Verification items for the finished model (mm, model axes). A direction names the side the tool comes from. Coordinates: 2 decimals unless noted, no trailing zeros. Order: outer loops, then holes, each group sorted by start corner. A loop starts at its lowest first (then second) coordinate and runs counter-clockwise, first axis right, second up. Notation, with made-up numbers: (-14.5, 21) - (36.5, 21) arc R12 cw to (36.5, 27) - close; hole circle Ø5 at (-1.5, 42). An arc over 180 degrees is marked (long way). One line per question, with ' | ' between items. Start each with the question number.
from build123d import *

# Parameters (mm, degrees)
SKETCH1_W               = 22.65
SKETCH1_H               = 31.12
PCB_DEPTH               = 1.3
SKETCH2_W               = 9.55
SKETCH2_H               = 7.3
IO_CONNECTOR_DEPTH      = 4.2
SKETCH3_W               = 3
SKETCH3_H               = 3.5
ANTENNA_CONNECTOR_DEPTH = 2
SKETCH15_W              = 3
SKETCH15_H              = 3.9
BUTTON_BASE_DEPTH       = 1.3
SKETCH16_R              = 0.9
BUTTON_TIP_DEPTH        = 0.8
SKETCH17_W              = 6.157933233
SKETCH17_H              = 6.029642957
SKETCH17_W_2            = 3.353874351
SKETCH17_H_2            = 3.005657888
SKETCH17_W_3            = 3.060639434
SKETCH17_H_3            = 1.576137673
SKETCH17_H_4            = 1.612792038
SKETCH17_W_4            = 3.201337113
SKETCH17_H_5            = 3.020980094
LOW_CHIPS_DEPTH         = 1
SKETCH18_W              = 6.492852738
SKETCH18_H              = 7.038252368
HIGH_CHIPS_DEPTH        = 2.7
SKETCH23_W              = 2
SKETCH23_H              = 0.8
LEDS_DEPTH              = 0.5
CORNERS_R               = 1
CUT_EXTRUDE1_REACH      = 24.031
SKETCH24_W              = 1.1
SKETCH24_H              = 2.5


with BuildPart() as part:
    # Sketch1 → PCB (new body)
    with BuildSketch(Plane(origin=(0, 0, 0), x_dir=(1, 0, 0), z_dir=(0, 1, 0))):
        Rectangle(SKETCH1_W, SKETCH1_H)
    extrude(amount=PCB_DEPTH)

    # Sketch2 → IO connector (add)
    with BuildSketch(Plane(origin=(0, 1.3, 0), x_dir=(1, 0, 0), z_dir=(0, 1, 0))):
        with Locations((6.55, -14.41)):
            Rectangle(SKETCH2_W, SKETCH2_H)
    extrude(amount=IO_CONNECTOR_DEPTH)

    # Sketch3 → Antenna connector (add)
    with BuildSketch(Plane(origin=(0, 1.3, 0), x_dir=(1, 0, 0), z_dir=(0, 1, 0))):
        with Locations((-8.025, 13.81)):
            Rectangle(SKETCH3_W, SKETCH3_H)
    extrude(amount=ANTENNA_CONNECTOR_DEPTH)

    # Sketch15 → Button base (add)
    with BuildSketch(Plane(origin=(0, 1.3, 0), x_dir=(1, 0, 0), z_dir=(0, 1, 0))):
        with Locations((-9.325, -12.41)):
            Rectangle(SKETCH15_W, SKETCH15_H)
    extrude(amount=BUTTON_BASE_DEPTH)

    # Sketch16 → Button tip (add)
    with BuildSketch(Plane(origin=(0, 2.6, 0), x_dir=(1, 0, 0), z_dir=(0, 1, 0))):
        with Locations(Location((-9.325, -12.41, 0), (0, 0, 90))):
            Circle(SKETCH16_R)
    extrude(amount=BUTTON_TIP_DEPTH)

    # Sketch17 → Low chips (add)
    with BuildSketch(Plane(origin=(0, 1.3, 0), x_dir=(1, 0, 0), z_dir=(0, 1, 0))):
        with Locations((-2.078363242, 3.759055692)):
            Rectangle(SKETCH17_W, SKETCH17_H)
        with Locations((-7.585681506, 8.185070203)):
            Rectangle(SKETCH17_W_2, SKETCH17_H_2)
        with Locations((9.825141625, 11.942142563)):
            Rectangle(SKETCH17_W_3, SKETCH17_H_3)
        with Locations((5.829815896, 11.044110633)):
            Rectangle(SKETCH17_W_3, SKETCH17_H_4)
        with Locations((-4.917111521, -2.959047528)):
            Rectangle(SKETCH17_W_4, SKETCH17_H_5)
    extrude(amount=LOW_CHIPS_DEPTH)

    # Sketch18 → High chips (add)
    with BuildSketch(Plane(origin=(0, 1.3, 0), x_dir=(1, 0, 0), z_dir=(0, 1, 0))):
        with Locations((8.086930252, -1.973636887)):
            Rectangle(SKETCH18_W, SKETCH18_H)
    extrude(amount=HIGH_CHIPS_DEPTH)

    # Sketch23 → LEDs (add)
    with BuildSketch(Plane(origin=(0, 1.3, 0), x_dir=(1, 0, 0), z_dir=(0, 1, 0))):
        with Locations((-9.725, -8.36)):
            Rectangle(SKETCH23_W, SKETCH23_H)
        with Locations((-9.725, -6.91)):
            Rectangle(SKETCH23_W, SKETCH23_H)
    extrude(amount=LEDS_DEPTH)

    # Corners
    corners_edges = [part.edges().sort_by_distance(p)[0] for p in [
        (11.325, 0.65, 15.56),
        (-11.325, 0.65, 15.56),
        (-11.325, 0.65, -15.56),
        (11.325, 0.65, -15.56),
    ]]
    fillet(corners_edges, radius=CORNERS_R)

    # Sketch24 → Cut-Extrude1 (cut, up to next)
    with BuildSketch(Plane(origin=(0, 5.5, 0), x_dir=(1, 0, 0), z_dir=(0, 1, 0)), mode=Mode.PRIVATE) as cut_extrude1_sk1:
        with Locations((10.775, -16.81)):
            Rectangle(SKETCH24_W, SKETCH24_H)
    cut_extrude1_tool1 = extrude(cut_extrude1_sk1.sketch, amount=-CUT_EXTRUDE1_REACH, mode=Mode.PRIVATE) & part.part
    # Sketch24 → Cut-Extrude1 (cut, up to next)
    with BuildSketch(Plane(origin=(0, 5.5, 0), x_dir=(1, 0, 0), z_dir=(0, 1, 0)), mode=Mode.PRIVATE) as cut_extrude1_sk2:
        with Locations((2.325, -16.81)):
            Rectangle(SKETCH24_W, SKETCH24_H)
    cut_extrude1_tool2 = extrude(cut_extrude1_sk2.sketch, amount=-CUT_EXTRUDE1_REACH, mode=Mode.PRIVATE) & part.part
    add(cut_extrude1_tool1.solids().sort_by_distance((10.775, 5.5, 16.81))[0], mode=Mode.SUBTRACT)
    add(cut_extrude1_tool2.solids().sort_by_distance((2.325, 5.5, 16.81))[0], mode=Mode.SUBTRACT)


solid = part.part
Item 1: Gauge pin test, flat ends, axial feed: pin 1 (6 mm diameter, centred on x = -2, z = 0.5, fed in from +Y); pin 2 (0.8 mm diameter, centred on y = 2, z = -12.5, fed in from -X) (3 decimals); pin 3 (1.2 mm diameter, centred on x = 6.5, z = 16.5, fed in from -Y). Record the tip position at first contact, or that the pin passes through.
Item 2: Mould release check, pull along Z, two halves, no side actions. Record for faces 4 (the flat face through (-2, 2, -6.774)), 5 (the flat face through (6, 2.3, -11)), 6 (the flat face through (8, 3, -1.545)): +Z half, -Z half, draft (parallel to the pull), parting line (faces both ways), or undercut.
Item 3: Set-up check for faces 1 (the flat face through (-5, 2.3, 3)), 2 (the flat face through (-6.518, 2, 3)), 3 (the flat face through (-5, 2, 1.449)): record each of +Z, -Z, +X, -X, +Y, -Y from which the full face is reachable in a straight line by a thin tool's end or side.
Item 4: Section check C-C (y = 4.9). Record the cut outline in (x, z) (3 decimals), then the cut area to 3 significant figures.
Item 5: Thickness scan on probe 1 along Z at (x, y) = (8.25, 3.05); probe 2 along Z at (x, y) = (-0.5, 1.05); probe 3 along X at (y, z) = (4.2, 13) (3 decimals). Record the ranges inside material, lowest first. Write a range as from..to.
Item 6: Section check D-D (z = 12.41). Record the cut outline in (x, y) (3 decimals), then the cut area to 3 significant figures.
Item 7: Section check B-B (x = 5.75). Record the cut outline in (y, z), then the cut area to 3 significant figures.
Item 8: Section check A-A (z = -6). Record the cut outline in (x, y) (3 decimals), then the cut area to 3 significant figures.
Completed:
1) pin 1: stops at y = 2.3 | pin 2: stops at x = -9.525 | pin 3: stops at y = 1.3
2) face 4: -Z half | face 5: draft | face 6: undercut
3) face 1: +Z, -Z, -X, +Y | face 2: +Z, -X, +Y | face 3: -X, +Y
4) outline: (1.775, 10.76) - (11.325, 10.76) - (11.325, 15.56) - (10.225, 15.56) - (10.225, 18.06) - (2.875, 18.06) - (2.875, 15.56) - (1.775, 15.56) - close | area: 64.2 mm^2
5) probe 1: z = -1.55..5.49, 10.76..18.06 | probe 2: z = -15.56..15.56 | probe 3: x = 1.775..11.325
6) outline: (-11.325, 0) - (11.325, 0) - (11.325, 5.5) - (1.775, 5.5) - (1.775, 1.3) - (-7.825, 1.3) - (-7.825, 2.6) - (-8.425, 2.6) - (-8.425, 3.4) - (-10.225, 3.4) - (-10.225, 2.6) - (-10.825, 2.6) - (-10.825, 1.3) - (-11.325, 1.3) - close | area: 74.9 mm^2
7) outline: (0, -15.56) - (1.3, -15.56) - (1.3, -11.85) - (2.3, -11.85) - (2.3, -10.24) - (1.3, -10.24) - (1.3, -1.55) - (4, -1.55) - (4, 5.49) - (1.3, 5.49) - (1.3, 10.76) - (5.5, 10.76) - (5.5, 18.06) - (1.3, 18.06) - (1.3, 15.56) - (0, 15.56) - close | area: 91.7 mm^2
8) outline: (-11.325, 0) - (11.325, 0) - (11.325, 1.3) - (1.001, 1.3) - (1.001, 2.3) - (-5.157, 2.3) - (-5.157, 1.3) - (-11.325, 1.3) - close | area: 35.6 mm^2
